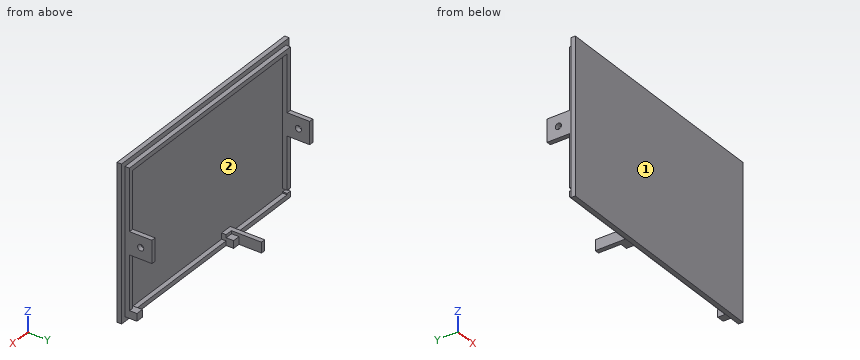
Autodesk Inventor part; units mm, degrees
ref_plane "Plano de trabalho1" through (-6.1, 6, -50.5) normal (-1, 0, 0) x (0, 0, 1)
ref_plane "Plano de trabalho2" through (-149.9, 6, -51.5) normal (1, 0, 0) x (0, 0, -1)
ref_plane "YZ Plane" through (0, 0, 0) normal (1, 0, 0) x (0, 1, 0)
sketch "Esboço6" plane through (0, 0, 0) normal (0, 1, 0) x (-1, 0, 0)
  line L0 (0, 0) -> (156, 0)
  line L1 (156, 0) -> (156, -103)
  line L2 (156, -103) -> (0, -103)
  line L3 (0, -103) -> (0, 0)
  dimension "d22" = 156
  dimension "d23" = 103
extrude "Extrusão4" add sketch "Esboço6" along normal blind 3
sketch "Esboço7" plane through (0, 3, 0) normal (0, 1, 0) x (1, 0, 0)
  line L0 (-152.9, 99.9) -> (-3.1, 99.9)
  line L1 (-3.1, 99.9) -> (-3.1, 3.1)
  line L2 (-3.1, 3.1) -> (-152.9, 3.1)
  line L3 (-152.9, 3.1) -> (-152.9, 99.9)
  line L4 (0, 0) -> (0, 103)
  line L5 (0, 103) -> (-156, 103)
  line L6 (-156, 103) -> (-156, 0)
  line L7 (-156, 0) -> (0, 0)
  line L8 (-149.9, 96.9) -> (-6.1, 96.9)
  line L9 (-6.1, 96.9) -> (-6.1, 6.1)
  line L10 (-6.1, 6.1) -> (-149.9, 6.1)
  line L11 (-149.9, 6.1) -> (-149.9, 96.9)
  dimension "d26" = 3.1
  dimension "d27" = 3.1
  dimension "d28" = 3.1
  dimension "d29" = 3.1
  dimension "d30" = 3
  dimension "d31" = 3
  dimension "d32" = 3
  dimension "d33" = 3
extrude "Extrusão5" add sketch "Esboço7" along normal blind 3 contours L0 L1 L2 L3
sketch "Esboço10" plane through (0, 6, 0) normal (0, 1, 0) x (1, 0, 0)
  line L0 (-3.1, 99.9) -> (-3.1, 3.1)
  line L1 (-3.1, 99.9) -> (-8.1, 99.9)
  line L2 (-8.1, 99.9) -> (-8.1, 94.9)
  line L3 (-8.1, 94.9) -> (-3.1, 94.9)
  line L4 (-3.1, 94.9) -> (-3.1, 99.9)
  line L5 (-152.9, 99.9) -> (-3.1, 99.9)
  line L6 (-93.1, 99.9) -> (-101.1, 99.9)
  line L7 (-101.1, 99.9) -> (-101.1, 94.9)
  line L8 (-101.1, 94.9) -> (-93.1, 94.9)
  line L9 (-93.1, 94.9) -> (-93.1, 99.9)
  point P0 (0, 0)
  dimension "d36" = 5
  dimension "d37" = 5
  dimension "d38" = 85
  dimension "d39" = 8
  dimension "d40" = 5
extrude "Extrusão6" add sketch "Esboço10" along normal blind 5 and the other way blind 6
sketch "Esboço13" plane through (-101.1, 3, -94.9) normal (0, 0, 1) x (1, 0, 0)
  line L0 (93, 3) -> (8, 3)
  line L1 (8, 3) -> (0, 3)
  line L2 (0, 3) -> (0, 23)
  line L3 (0, 23) -> (3, 23)
  line L4 (3, 23) -> (3, 8)
  line L5 (8, 8) -> (0, 8)
  line L6 (3, 8) -> (8, 8)
  line L7 (8, 8) -> (8, 3)
  point P0 (101.1, -3)
  dimension "d45" = 8
  dimension "d46" = 20
  dimension "d47" = 3
extrude "Extrusão7" add sketch "Esboço13" against normal blind 5 contours L2 L3 L4 L5
sketch "Esboço14" plane through (-101.1, 3, -94.9) normal (0, 0, 1) x (1, 0, 0)
  line L0 (0, 3) -> (0, 23)
  line L1 (0, 23) -> (3, 23)
  line L2 (0, 23) -> (3, 23)
  line L3 (-54.9, -3) -> (101.1, -3)
  line L4 (0, 0) -> (0, 23)
  line L5 (0, 0) -> (8, 0)
  line L6 (-51.8, 0) -> (98, 0)
  line L7 (8, 0) -> (8, 3)
  line L8 (93, 3) -> (8, 3)
  line L9 (8, 3) -> (3, 3)
  line L10 (3, 3) -> (3, 23)
  line L11 (3, 23) -> (3, 8)
  line L12 (8, 8) -> (3, 8)
  dimension "d53" = 8
  dimension "d54" = 5
  dimension "d55" = 5
extrude "Extrusão8" add sketch "Esboço14" along normal blind 2
ref_plane "Plano de trabalho1" through (-6.1, 6, -50.5) normal (-1, 0, 0) x (0, 0, 1)
ref_plane "Plano de trabalho2" through (-149.9, 6, -51.5) normal (1, 0, 0) x (0, 0, -1)
sketch "Esboço18" plane through (-6.1, 6, -50.5) normal (-1, 0, 0) x (0, 0, 1)
  line L0 (6.5, 0) -> (-8.5, 0)
  line L1 (-8.5, 0) -> (-8.5, 15)
  line L2 (-8.5, 15) -> (6.5, 15)
  line L3 (6.5, 15) -> (6.5, 0)
  line L4 (-49.4, 0) -> (47.4, 0)
  line L5 (47.4, -3) -> (47.4, 0)
  dimension "d67" = 15
  dimension "d68" = 15
  dimension "d71" = 40.9
extrude "Extrusão9" add sketch "Esboço18" against normal blind 3
sketch "Esboço19" plane through (-149.9, 6, -51.5) normal (1, 0, 0) x (0, 0, -1)
  line L0 (-7.5, 0) -> (7.5, 0)
  line L1 (7.5, 0) -> (7.5, 15)
  line L2 (7.5, 15) -> (-7.5, 15)
  line L3 (-7.5, 15) -> (-7.5, 0)
  line L4 (48.4, -3) -> (48.4, 0)
  line L5 (48.4, 0) -> (-48.4, 0)
  point P0 (-51.5, -6)
  dimension "d72" = 15
  dimension "d73" = 15
  dimension "d74" = 40.9
extrude "Extrusão10" add sketch "Esboço19" against normal blind 3
sketch "Esboço21" plane through (-152.9, 3, -99.9) normal (-1, 0, 0) x (0, 0, 1)
  circle A0 centre (48.4, 10.5) radius 2.05
  line L0 (55.9, 3) -> (55.9, 18)
  line L1 (55.9, 18) -> (40.9, 18)
  dimension "d87" = 7.5
  dimension "d88" = 7.5
  dimension "d89" = 4.1
extrude "Extrusão13" cut sketch "Esboço21" against normal through all
sketch "Esboço22" plane through (-152.9, 3, -99.9) normal (-1, 0, 0) x (0, 0, 1)
  line L0 (5, 3) -> (40.9, 3)
  line L1 (99.9, 0) -> (-3.1, 0)
  line L2 (5.9, 3) -> (3.9, 3)
  line L3 (3.9, 3) -> (3.9, 0)
  line L4 (3.9, 0) -> (5.9, 0)
  line L5 (5.9, 0) -> (5.9, 3)
  line L6 (-3.1, -3) -> (-3.1, 0)
  dimension "d92" = 2
  dimension "d93" = 7
extrude "Extrusão14" cut sketch "Esboço22" against normal blind 10
properties part number "Encaixe"
Could you check a few things on this model? Use its own coordinates, in mm. Face numbers are marked on the shaded views. Round coordinates to 2 decimals unless told otherwise and drop trailing zeros. Order: outer loops, then holes, each group sorted by start corner. A loop starts at its lowest first (then second) coordinate and runs counter-clockwise, first axis right, second up.
(1) I'm going to push flat-ended pins straight in: pin 1 (1.5 mm diameter, centred on x = -151, y = 5, fed in from +Z); pin 2 (10 mm diameter, centred on x = -71, z = -12.5, fed in from -Y); pin 3 (2.5 mm diameter, centred on x = -151.5, z = -81, fed in from +Y); pin 4 (3.5 mm diameter, centred on x = -4, y = 16.5, fed in from +Z). Where does each tip first touch, or does it pass through?
Response values:
pin 1: stops at z = -3.1
pin 2: stops at y = 0
pin 3: stops at y = 6
pin 4: stops at z = -44
(2) Imagine slicing it at C-C (x = -19.5). Write out the boundary of the cut face in (y, z).
Response values:
outline: (0, -103) - (3, -103) - (3, -99.9) - (6, -99.9) - (6, -96.9) - (3, -96.9) - (3, -6.1) - (6, -6.1) - (6, -3.1) - (3, -3.1) - (3, 0) - (0, 0) - close
(3) If we mould it in two halves opening along Z, with no side actions, what happens to the marked faces 1 and 2? For each: released by +Z, released by -Z, zero draft, split by the parting line, or undercut.
Response values:
face 1: zero draft
face 2: undercut
(4) Please list where these lines run through material, in increasing order: line 1 along X through (y, z) = (4.5, -70); line 2 along Y through (x, z) = (-5.2, -51.5); line 3 along Z through (x, y) = (-113.5, 5).
Response values:
line 1: x = -152.9 to -149.9, -6.1 to -3.1
line 2: y = 0 to 11.45, 15.55 to 21
line 3: z = -99.9 to -96.9, -6.1 to -3.1
(5) Imagine slicing it at A-A (y = 13.5). Write out the boundary of the cut face in (x, z).
Response values:
outline: (-152.9, -59) - (-149.9, -59) - (-149.9, -53.55) - (-152.9, -53.55) - close; (-152.9, -49.45) - (-149.9, -49.45) - (-149.9, -44) - (-152.9, -44) - close; (-101.1, -99.9) - (-98.1, -99.9) - (-98.1, -92.9) - (-101.1, -92.9) - close; (-6.1, -59) - (-3.1, -59) - (-3.1, -53.55) - (-6.1, -53.55) - close; (-6.1, -49.45) - (-3.1, -49.45) - (-3.1, -44) - (-6.1, -44) - close
(6) Imagine slicing it at D-D (z = -24). Write out the boundary of the cut face in (x, y).
Response values:
outline: (-156, 0) - (0, 0) - (0, 3) - (-3.1, 3) - (-3.1, 6) - (-6.1, 6) - (-6.1, 3) - (-149.9, 3) - (-149.9, 6) - (-152.9, 6) - (-152.9, 3) - (-156, 3) - close
(7) Imagine slicing it at B-B (z = -51.5). Write out the boundary of the cut face in (x, y).
Response values:
outline: (-156, 0) - (0, 0) - (0, 3) - (-3.1, 3) - (-3.1, 11.45) - (-6.1, 11.45) - (-6.1, 3) - (-149.9, 3) - (-149.9, 11.45) - (-152.9, 11.45) - (-152.9, 3) - (-156, 3) - close; (-152.9, 15.55) - (-149.9, 15.55) - (-149.9, 21) - (-152.9, 21) - close; (-6.1, 15.55) - (-3.1, 15.55) - (-3.1, 21) - (-6.1, 21) - close
